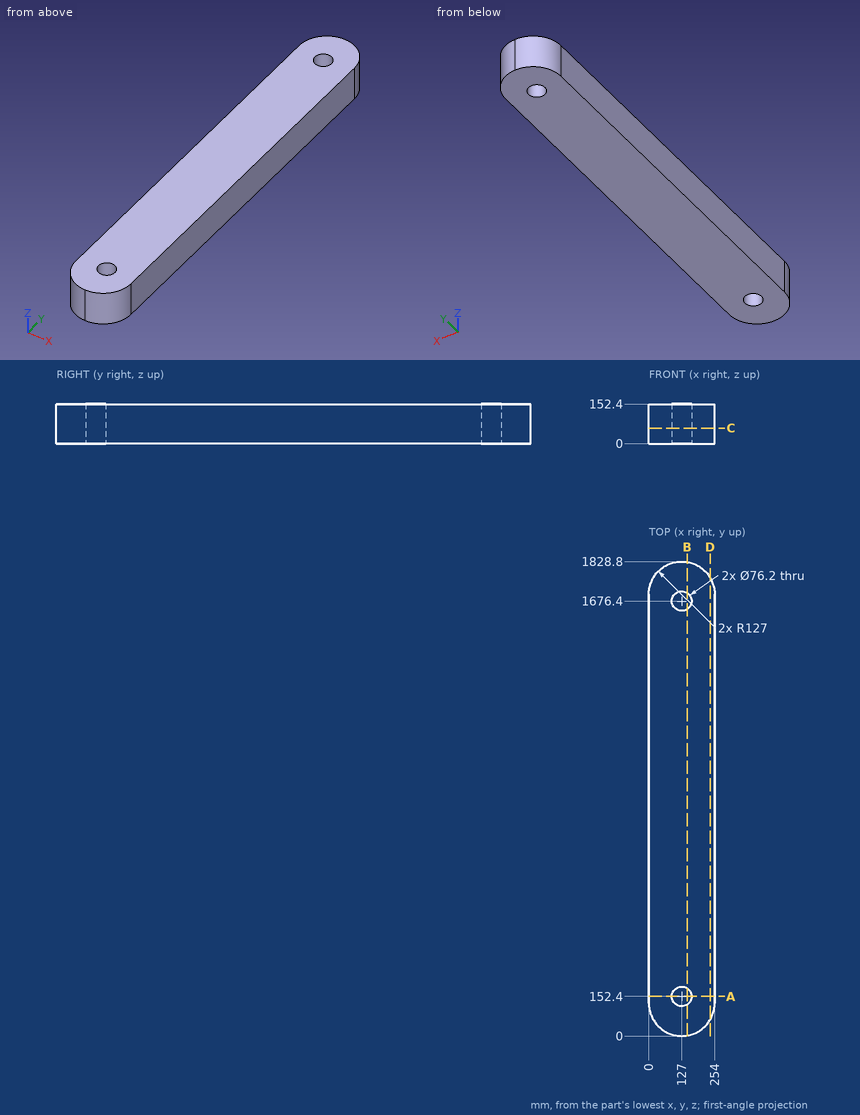
Design review of the part shown in the three views and the two pictorial views. Dimensions are in mm from the part's minimum x, y and z. Give positions to 0.01 mm unless a question says otherwise; leave off trailing zeros. Write each loop counter-clockwise with the first axis right and the second up, starting at its lowest first coordinate (ties: lowest second). Pieces come first, ordered by that corner, then holes. Notation, with made-up numbers: M 17,29.25 L 72,29.25 A15 ccw 72,44.25 Z; hole C 28.5,-5 d3. An arc over 180 degrees is marked long. One line per question, with ' | ' between items. Start each with the question number.
Item 1: We need section B-B on x = 147.5. Write out the cut boundary in (y, z).
Item 2: Wall thickness on line 1 (X direction, y = 1676, z = 56); line 2 (X direction, y = 1648, z = 105.5); line 3 (Y direction, x = 107.5, z = 91): over which ranges is each line inside the solid? List them lowest first. Write a range as from..to.
Item 3: We need section C-C on z = 59. Give the number of separate pieces and of enclosed holes in the cut face, plus the area to 3 significant figures.
Item 4: For pin 1 (6 mm diameter, centred on x = 93.5, z = 45, fed in from -Y), flat-tipped, find the tip position at first contact; note if it passes through.
Item 5: We need section D-D on x = 236. Write out the cut boundary in (y, z), plus the area to 3 significant figures.
Item 6: We need section A-A on y = 152.4. Write out the cut boundary in (x, z), plus the area to 3 significant figures.
Results found:
1) outline: M 1.67,0 L 120.29,0 L 120.29,152.4 L 1.67,152.4 Z; M 184.51,0 L 1644.29,0 L 1644.29,152.4 L 184.51,152.4 Z; M 1708.51,0 L 1827.13,0 L 1827.13,152.4 L 1708.51,152.4 Z
2) line 1: x = 0..88.9, 165.1..254 | line 2: x = 0..101.6, 152.4..254 | line 3: y = 1.51..119.67, 185.13..1643.67, 1709.13..1827.29
3) separate pieces: 1 | enclosed holes: 2 | area: 442,000 mm2
4) pin 1: stops at y = 3.72
5) outline: M 61.82,0 L 1766.98,0 L 1766.98,152.4 L 61.82,152.4 Z | area: 260,000 mm2
6) outline: M 0,0 L 88.9,0 L 88.9,152.4 L 0,152.4 Z; M 165.1,0 L 254,0 L 254,152.4 L 165.1,152.4 Z | area: 27,100 mm2
